For this review, take the finished solid that the model builds, in its own axes (mm). A direction names the side the tool comes from. Give positions to 0.01 mm unless a question says otherwise; leave off trailing zeros. Write each loop counter-clockwise with the first axis right and the second up, starting at its lowest first coordinate (ties: lowest second). Pieces come first, ordered by that corner, then holes. Notation, with made-up numbers: (17.5, 51.5) -> (21.5, 51.5) arc R31 cw to (21.5, 83.5) -> close; hole circle Ø1 at (42.5, -37.5). An arc over 180 degrees is marked (long way). Return JSON: item names as keys, results as strings.
from build123d import *

# Parameters (mm, degrees)
SKETCH_2_R          = 100
SKETCH_2_R_2        = 3
SKETCH_2_R_3        = 30
EXTRUDE_1_DEPTH     = 20
SKETCH_3_R          = 43
CUT_EXTRUDE_1_DEPTH = 11


with BuildPart() as part:
    # 草图2 → 凸台-拉伸1 (new body)
    with BuildSketch(Plane(origin=(0, 0, 0), x_dir=(1, 0, 0), z_dir=(0, 1, 0))):
        with Locations(Location((0, 0, 0), (0, 0, 270))):
            Circle(SKETCH_2_R)
        with Locations(Location((0, 90, 0), (0, 0, 270))):
            Circle(SKETCH_2_R_2, mode=Mode.SUBTRACT)
        with Locations(Location((90, 0, 0), (0, 0, 270))):
            Circle(SKETCH_2_R_2, mode=Mode.SUBTRACT)
        with Locations(Location((0, -90, 0), (0, 0, 270))):
            Circle(SKETCH_2_R_2, mode=Mode.SUBTRACT)
        with Locations(Location((-90, 0, 0), (0, 0, 270))):
            Circle(SKETCH_2_R_2, mode=Mode.SUBTRACT)
        with Locations(Location((0, 0, 0), (0, 0, 270))):
            Circle(SKETCH_2_R_3, mode=Mode.SUBTRACT)
    extrude(amount=EXTRUDE_1_DEPTH)

    # 草图3 → 切除-拉伸1 (cut)
    with BuildSketch(Plane.XZ):
        with Locations(Location((0, 0, 0), (0, 0, 270))):
            Circle(SKETCH_3_R)
    extrude(amount=-CUT_EXTRUDE_1_DEPTH, mode=Mode.SUBTRACT)


solid = part.part
1. The part is to be moulded in two halves that separate along Z. For faces 3 (the flat face through (24, 20, 21)), 4 (the flat face through (29, 11, -9)), 5 (the cylindrical face through (30.04, 9.86, 95.38)), 6 (the cylindrical face through (-92.93, 9.86, -0.65)), say which applies: +Z half, -Z half, draft (parallel to the pull), parting line (faces both ways), or undercut.
Results found:
{"face 3": "draft", "face 4": "undercut", "face 5": "parting line", "face 6": "undercut"}
2. Add section D-D, the plane z = 90. State the section outline as (x, y) points, plus the area to 3 significant figures.
Results found:
{"outline": "(-43.59, 0) -> (-3, 0) -> (-3, 20) -> (-43.59, 20) -> close; (3, 0) -> (43.59, 0) -> (43.59, 20) -> (3, 20) -> close", "area": "1,620 mm²"}
3. Add section C-C, the plane x = -90. State the section outline as (y, z) points.
Results found:
{"outline": "(0, -43.59) -> (20, -43.59) -> (20, -3) -> (0, -3) -> close; (0, 3) -> (20, 3) -> (20, 43.59) -> (0, 43.59) -> close"}
4. To check wall thickness, follow probe 1 along X at (y, z) = (16, 0.5); probe 2 along X at (y, z) = (9.25, 0); probe 3 along Y at (x, z) = (19, -27.5). State the ranges of each line that lie inside material, in increasing order.
Results found:
{"probe 1": "x = -100 to -92.96, -87.04 to -30, 30 to 87.04, 92.96 to 100", "probe 2": "x = -100 to -93, -87 to -43, 43 to 87, 93 to 100", "probe 3": "y = 11 to 20"}
5. For pin 1 (3 mm diameter, centred on x = 68, y = 13, fed in from +Z); pin 2 (2 mm diameter, centred on x = 68.5, y = 5.5, fed in from +Z); pin 3 (1.5 mm diameter, centred on x = 39, y = 11, fed in from -Z); pin 4 (8 mm diameter, centred on x = 0, z = 90, fed in from -Y), all flat-tipped, find the tip position at first contact; note any pin that passes through.
Results found:
{"pin 1": "stops at z = 74.68", "pin 2": "stops at z = 73.78", "pin 3": "stops at z = -92.4", "pin 4": "stops at y = 0"}
6. For faces 1 (the cylindrical face through (0, 10, -93)), 2 (the cylindrical face through (29.061, 5.423, 31.693)), list the 3-axis set-ups (+Z, -Z, +X, -X, +Y, -Y) from which the entire face can be reached by the end or side of a thin tool; tool diameter is ignored.
Results found:
{"face 1": "+Y, -Y", "face 2": "-Y"}
7. Add section A-A, the plane z = 0. State the section outline as (x, y) points.
Results found:
{"outline": "(-100, 0) -> (-93, 0) -> (-93, 20) -> (-100, 20) -> close; (-87, 0) -> (-43, 0) -> (-43, 11) -> (-30, 11) -> (-30, 20) -> (-87, 20) -> close; (30, 11) -> (43, 11) -> (43, 0) -> (87, 0) -> (87, 20) -> (30, 20) -> close; (93, 0) -> (100, 0) -> (100, 20) -> (93, 20) -> close"}
8. Add section B-B, the plane x = 0. State the section outline as (y, z) points.
Results found:
{"outline": "(0, -100) -> (20, -100) -> (20, -93) -> (0, -93) -> close; (0, -87) -> (20, -87) -> (20, -30) -> (11, -30) -> (11, -43) -> (0, -43) -> close; (0, 43) -> (11, 43) -> (11, 30) -> (20, 30) -> (20, 87) -> (0, 87) -> close; (0, 93) -> (20, 93) -> (20, 100) -> (0, 100) -> close"}
